Here's how the part is built. I have some questions about the finished solid (model axes, mm). A direction names the side the tool comes from. Round coordinates to 2 decimals unless told otherwise and drop trailing zeros. Order: outer loops, then holes, each group sorted by start corner. A loop starts at its lowest first (then second) coordinate and runs counter-clockwise, first axis right, second up. Notation, with made-up numbers: (88, 78.25) - (119, 78.25) arc R25 cw to (119, 111.25) - close; hole circle Ø9 at (28, -12.75). An arc over 180 degrees is marked (long way). Answer as a JSON object with one key per item and string values.
```python
from build123d import *

# Parameters (mm, degrees)
BOSS_EXTRUDE1_DEPTH = 15
SKETCH2_W           = 21
SKETCH2_H           = 8
SKETCH2_W_2         = 17
SKETCH2_H_2         = 17
CUT_EXTRUDE2_DEPTH  = 6
SKETCH3_R           = 5
CUT_EXTRUDE3_DEPTH  = 10
BOSS_EXTRUDE3_DEPTH = 15
SKETCH5_R           = 3.5
BOSS_EXTRUDE4_DEPTH = 4
CHAMFER1_SIZE       = 15
FILLET1_R           = 5


with BuildPart() as part:
    # Sketch1 → Boss-Extrude1 (new body)
    with BuildSketch(Plane(origin=(0, 0, 0), x_dir=(1, 0, 0), z_dir=(0, 1, 0))):
        with BuildLine():
            Line((-6, -26.842412903), (40.363636364, 15.657587097))
            Line((40.363636364, 15.657587097), (47.363636364, 15.657587097))
            ThreePointArc((47.363636364, 15.657587097), (54.863636364, 28.157587097), (47.363636364, 40.657587097))
            Line((47.363636364, 40.657587097), (40.363636364, 40.657587097))
            Line((40.363636364, 40.657587097), (-6, 83.157587097))
            Line((-6, 83.157587097), (-6, -26.842412903))
        make_face()
    extrude(amount=BOSS_EXTRUDE1_DEPTH)

    # Sketch2 → Cut-Extrude2 (cut)
    with BuildSketch(Plane.XZ):
        with Locations((20, -28.157587097)):
            Rectangle(SKETCH2_W, SKETCH2_H)
        with Locations((39, -28.157587097)):
            Rectangle(SKETCH2_W_2, SKETCH2_H_2)
    extrude(amount=-CUT_EXTRUDE2_DEPTH, mode=Mode.SUBTRACT)

    # Sketch3 → Cut-Extrude3 (cut, through all)
    with BuildSketch(Plane(origin=(0, 6, 0), x_dir=(-1, 0, 0), z_dir=(0, 1, 0))):
        with Locations((-39, -28.157587097)):
            Circle(SKETCH3_R)
    extrude(amount=CUT_EXTRUDE3_DEPTH, mode=Mode.SUBTRACT)

    # Sketch6 → Boss-Extrude3 (add)
    with BuildSketch(Plane.XZ):
        with BuildLine():
            Line((-6, 26.842412903), (-6, -83.157587097))
            Line((-6, -83.157587097), (16.563859252, -62.474049449))
            ThreePointArc((16.563859252, -62.474049449), (-2, -28.157587097), (16.563859252, 6.158875255))
            Line((16.563859252, 6.158875255), (-6, 26.842412903))
        make_face()
    extrude(amount=BOSS_EXTRUDE3_DEPTH)

    # Sketch5 → Boss-Extrude4 (add)
    with BuildSketch(Plane.ZY.offset(6)):
        with Locations((-53.157587097, -8)):
            Circle(SKETCH5_R)
        with Locations((-3.157587097, -8)):
            Circle(SKETCH5_R)
    extrude(amount=BOSS_EXTRUDE4_DEPTH)

    # Chamfer1
    chamfer1_edges = [part.edges().sort_by_distance(p)[0] for p in [
        (-6, 15, -28.157587097),
    ]]
    chamfer(chamfer1_edges, length=CHAMFER1_SIZE)

    # Fillet1
    fillet1_edges = [part.edges().sort_by_distance(p)[0] for p in [
        (43.863636364, 15, -40.657587097),
        (47.363636364, 7.5, -15.657587097),
        (40.363636364, 7.5, -15.657587097),
        (40.363636364, 7.5, -40.657587097),
        (47.363636364, 7.5, -40.657587097),
        (24.681818182, 15, -55.032587097),
        (43.863636364, 15, -15.657587097),
        (54.863636364, 15, -28.157587097),
        (24.681818182, 15, -1.282587097),
        (9, 15, -28.157587097),
    ]]
    fillet(fillet1_edges, radius=FILLET1_R)


solid = part.part
```
1. Imagine slicing it at A-A (y = -8). List the corners of the cut face in (x, z) for me.
Responses:
{"outline": "(-10, -56.66) - (-6, -56.66) - (-6, -83.16) - (16.56, -62.47) arc R41 cw to (16.56, 6.16) - (-6, 26.84) - (-6, 0.34) - (-10, 0.34) - (-10, -6.66) - (-6, -6.66) - (-6, -49.66) - (-10, -49.66) - close"}
2. Thinking about a two-plate mould opening in Z: for faces 5 (the face through (44, 5, -40.658)), 6 (the face through (-1.996, -7.395, -28.727)), 7 (the face through (54.862, 4.93, -27.968)), which applies, pulls with the +Z half, pulls with the -Z half, needs draft (parallel to the pull), parting line crosses it, or undercut?
Responses:
{"face 5": "pulls with the -Z half", "face 6": "undercut", "face 7": "parting line crosses it"}
3. For faces 1 (the face through (44.164, 13.574, -17.161)), 2 (the face through (-7.972, -11.417, -3.916)), 3 (the face through (30.5, 3, -34)), 4 (the face through (44, 5, -15.658)), which set-ups out of +Z, -Z, +X, -X, +Y, -Y let a thin tool reach every point of the face, with its end or its side?
Responses:
{"face 1": "+Z, +X, +Y", "face 2": "-X", "face 3": "-Y", "face 4": "+Z, +X, +Y, -Y"}
4. If I drill on L1, parallel to Z at x = 45.5, y = 1.5; L2, parallel to Z at x = 39, y = 8.5; L3, parallel to Y at x = 12, z = -27, over which ranges is the centre line in solid material (lowest first)? Write a range as [from, to].
Responses:
{"L1": "[-40.66, -36.66], [-19.66, -15.66]", "L2": "[-41.91, -33.16], [-23.16, -14.41]", "L3": "[6, 15]"}
5. Imagine slicing it at B-B (y = 3). List the corners of the cut face in (x, z) for me.
Responses:
{"outline": "(-3, -80.41) - (38.93, -41.97) arc R5 cw to (42.31, -40.66) - (45.97, -40.66) arc R5 ccw to (48.84, -39.75) arc R14.17 ccw to (48.84, -16.57) arc R5 ccw to (45.97, -15.66) - (42.31, -15.66) arc R5 cw to (38.93, -14.34) - (-3, 24.09) - close; hole (9.5, -32.16) - (30.5, -32.16) - (30.5, -36.66) - (47.5, -36.66) - (47.5, -19.66) - (30.5, -19.66) - (30.5, -24.16) - (9.5, -24.16) - close"}
6. For P1, Ø1, axis at y = -6, z = -49.5, coming from the +X side; P2, Ø12, axis at x = 45, y = -1.5, coming from the +Z side; P3, Ø3, axis at x = 17.5, y = 4, coming from the -Z side, each with a flat end and sliding along its axis, tell me the tip position at first contact or that it passes through.
Responses:
{"P1": "x = 4.3", "P2": "z = -14.57", "P3": "z = -62.99"}
